Part model, mm, in its own coordinate system. Give positions to 0.01 mm unless a question says otherwise; leave off trailing zeros. Loops run counter-clockwise (first coordinate to the right, second up) from the corner with the lowest first, then second, coordinate; pieces in that order, holes last. Notation, with made-up numbers: (-1.5, 1) -> (25.5, 1) arc R25 ccw to (25.5, 33) -> close; hole circle Ø10 at (-1, -14). An arc over 180 degrees is marked (long way). Write item = value, one per line.
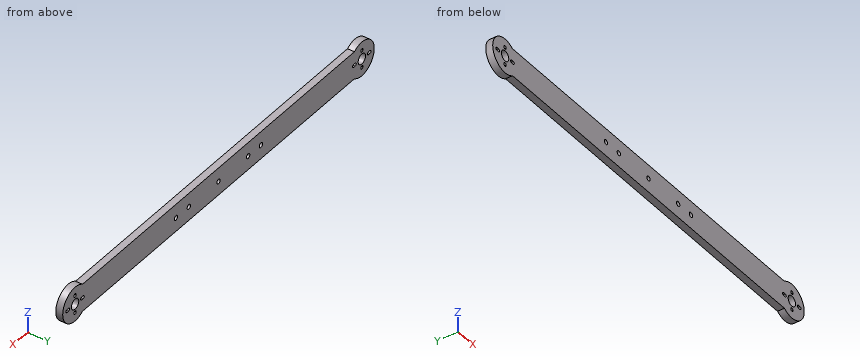
from build123d import *

# Parameters (mm, degrees)
BOSS_EXTRUDE1_DEPTH = 6.35
SKETCH2_R           = 4.75
CUT_EXTRUDE1_DEPTH  = 201.754423986
SKETCH3_R           = 2.159
CUT_EXTRUDE2_DEPTH  = 201.754423986
SKETCH4_R           = 2.159
CUT_EXTRUDE3_DEPTH  = 201.754423986


with BuildPart() as part:
    # Sketch1 → Boss-Extrude1 (new body)
    with BuildSketch(Plane(origin=(0, 0, 0), x_dir=(1, 0, 0), z_dir=(0, 1, 0))):
        with BuildLine():
            Line((-174.625, 12.7), (174.625, 12.7))
            ThreePointArc((174.625, 12.7), (200.025, 0), (174.625, -12.7))
            Line((174.625, -12.7), (-174.625, -12.7))
            ThreePointArc((-174.625, -12.7), (-200.025, 0), (-174.625, 12.7))
        make_face()
    extrude(amount=BOSS_EXTRUDE1_DEPTH)

    # Sketch2 → Cut-Extrude1 (cut, through all)
    with BuildSketch(Plane(origin=(0, 6.35, 0), x_dir=(1, 0, 0), z_dir=(0, 1, 0))):
        with Locations(Location((184.15, 0, 0), (0, 0, 270))):
            Circle(SKETCH2_R)
        with Locations(Location((-184.15, 0, 0), (0, 0, 90))):
            Circle(SKETCH2_R)
        with BuildLine():
            Line((173.691383345, 1.375), (175.608616655, 1.375))
            ThreePointArc((175.608616655, 1.375), (176.983616655, 0), (175.608616655, -1.375))
            Line((175.608616655, -1.375), (173.691383345, -1.375))
            ThreePointArc((173.691383345, -1.375), (172.316383345, 0), (173.691383345, 1.375))
        make_face()
        with BuildLine():
            Line((194.608616655, 1.375), (192.691383345, 1.375))
            ThreePointArc((192.691383345, 1.375), (191.316383345, 0), (192.691383345, -1.375))
            Line((192.691383345, -1.375), (194.608616655, -1.375))
            ThreePointArc((194.608616655, -1.375), (195.983616655, 0), (194.608616655, 1.375))
        make_face()
        with BuildLine():
            Line((185.525, 8.25), (185.525, 7.75))
            ThreePointArc((185.525, 7.75), (184.15, 6.375), (182.775, 7.75))
            Line((182.775, 7.75), (182.775, 8.25))
            ThreePointArc((182.775, 8.25), (184.15, 9.625), (185.525, 8.25))
        make_face()
        with BuildLine():
            Line((185.525, -8.25), (185.525, -7.75))
            ThreePointArc((185.525, -7.75), (184.15, -6.375), (182.775, -7.75))
            Line((182.775, -7.75), (182.775, -8.25))
            ThreePointArc((182.775, -8.25), (184.15, -9.625), (185.525, -8.25))
        make_face()
        with BuildLine():
            Line((-185.525, -8.25), (-185.525, -7.75))
            ThreePointArc((-185.525, -7.75), (-184.15, -6.375), (-182.775, -7.75))
            Line((-182.775, -7.75), (-182.775, -8.25))
            ThreePointArc((-182.775, -8.25), (-184.15, -9.625), (-185.525, -8.25))
        make_face()
        with BuildLine():
            Line((-185.525, 8.25), (-185.525, 7.75))
            ThreePointArc((-185.525, 7.75), (-184.15, 6.375), (-182.775, 7.75))
            Line((-182.775, 7.75), (-182.775, 8.25))
            ThreePointArc((-182.775, 8.25), (-184.15, 9.625), (-185.525, 8.25))
        make_face()
        with BuildLine():
            Line((-194.608616655, 1.375), (-192.691383345, 1.375))
            ThreePointArc((-192.691383345, 1.375), (-191.316383345, 0), (-192.691383345, -1.375))
            Line((-192.691383345, -1.375), (-194.608616655, -1.375))
            ThreePointArc((-194.608616655, -1.375), (-195.983616655, 0), (-194.608616655, 1.375))
        make_face()
        with BuildLine():
            Line((-173.691383345, 1.375), (-175.608616655, 1.375))
            ThreePointArc((-175.608616655, 1.375), (-176.983616655, 0), (-175.608616655, -1.375))
            Line((-175.608616655, -1.375), (-173.691383345, -1.375))
            ThreePointArc((-173.691383345, -1.375), (-172.316383345, 0), (-173.691383345, 1.375))
        make_face()
    extrude(amount=-CUT_EXTRUDE1_DEPTH, mode=Mode.SUBTRACT)

    # Sketch3 → Cut-Extrude2 (cut, through all)
    with BuildSketch(Plane(origin=(0, 6.35, 0), x_dir=(1, 0, 0), z_dir=(0, 1, 0))):
        with Locations(Location((0, 0, 0), (0, 0, 270))):
            Circle(SKETCH3_R)
        with Locations(Location((38.1, 0, 0), (0, 0, 270))):
            Circle(SKETCH3_R)
        with Locations(Location((-38.1, 0, 0), (0, 0, 270))):
            Circle(SKETCH3_R)
    extrude(amount=-CUT_EXTRUDE2_DEPTH, mode=Mode.SUBTRACT)

    # Sketch4 → Cut-Extrude3 (cut, through all)
    with BuildSketch(Plane(origin=(0, 6.35, 0), x_dir=(1, 0, 0), z_dir=(0, 1, 0))):
        with Locations(Location((54.61, 0, 0), (0, 0, 270))):
            Circle(SKETCH4_R)
        with Locations(Location((-54.61, 0, 0), (0, 0, 90))):
            Circle(SKETCH4_R)
    extrude(amount=-CUT_EXTRUDE3_DEPTH, mode=Mode.SUBTRACT)


solid = part.part
1) Drill centre lines: line 1 along Z through (x, y) = (-184.15, 4.5) (3 decimals); line 2 along X through (y, z) = (5.5, 3); line 3 along X through (y, z) = (4.25, -8.5). Where is each one in solid material? Low to high. Write a range as [from, to].
Resolved:
line_1 = [-15.875, -9.625], [-6.375, -4.75], [4.75, 6.375], [9.625, 15.875]
line_2 = [-199.74, -187.83], [-180.47, 180.47], [187.83, 199.74]
line_3 = [-197.56, -185.5], [-182.8, 182.8], [185.5, 197.56]
2) Slice it at B-B, the plane x = 115. List the corners of the cut face in (y, z).
Resolved:
outline = (0, -12.7) -> (6.35, -12.7) -> (6.35, 12.7) -> (0, 12.7) -> close
3) Slice it at A-A, the plane y = 1. Count the separate pieces of the cut face and the enclosed holes in it, and give its area (3 significant figures).
Resolved:
separate_pieces = 1
enclosed_holes = 15
area = 9,940 mm²
4) Drop flat-ended pins along their axis: P1, Ø2, axis at x = 174.5, y = 4, coming from the +Z side; P2, Ø1.5, axis at x = -175, y = 2, coming from the +Z side; P3, Ø3, axis at x = 25.5, y = 3.5, coming from the +Z side; P4, Ø7.5, axis at x = 184.15, z = 0, coming from the +Y side. Give the stop position or say it passes through.
Resolved:
P1 = 13.31
P2 = 13.47
P3 = 12.7
P4 = through
